The model under review builds one solid part; all positions refer to its coordinate system, in mm. A direction names the side the tool comes from. Coordinates: 2 decimals unless noted, no trailing zeros. Loops run counter-clockwise (first coordinate to the right, second up) from the corner with the lowest first, then second, coordinate; pieces in that order, holes last. Notation, with made-up numbers: M 51,61 L 88,61 A33 ccw 88,98 Z; hole C -28.75,-31.75 d2. An arc over 180 degrees is marked long. Use one line per item in the form item = value.
Autodesk Fusion 360 part; units mm, degrees
sketch "Sketch1" plane through (0, 0, 0) normal (0, 1, 0) x (1, 0, 0)
  line L0 (26, 0) -> (-26, 0)
  line L1 (0, 0) -> (0, -40) construction
  circle A0 centre (0, -20) radius 14
  circle A1 centre (0, -20) radius 19 construction
  line L2 (-26, 0) -> (-26, -28)
  line L3 (-26, -28) -> (-14, -40)
  line L4 (-14, -40) -> (14, -40)
  line L5 (14, -40) -> (26, -28)
  line L6 (26, -28) -> (26, 0)
  line L7 (26, -20) -> (-26, -20) construction
  line L8 (0, -20) -> (13.435, -33.435) construction
  line L9 (0, -20) -> (19, -20) construction
  line L10 (0, -20) -> (13.435, -6.565) construction
  line L11 (0, -20) -> (19, -20) construction
  line L12 (0, -20) -> (-13.435, -33.435) construction
  line L13 (0, -20) -> (19, -20) construction
  line L14 (0, -20) -> (-13.435, -6.565) construction
  line L15 (0, -20) -> (19, -20) construction
  circle A2 centre (-13.435, -33.435) radius 2.5
  circle A3 centre (-19, -20) radius 2.5
  circle A4 centre (-13.435, -6.565) radius 2.5
  circle A5 centre (13.435, -33.435) radius 2.5
  circle A6 centre (13.435, -6.565) radius 2.5
  circle A7 centre (19, -20) radius 2.5
  point P0 (0, -20)
  dimension "d2" = 52
  dimension "d3" = 40
  dimension "d4" = 28
  dimension "d5" = 38
  dimension "d6" = 135
  dimension "d8" = 135
  dimension "d10" = 12
  dimension "d12" = 45
  dimension "d13" = 45
  dimension "d16" = 45
  dimension "d17" = 45
  dimension "d18" = 5
  dimension "d19" = 5
  dimension "d20" = 5
  dimension "d21" = 5
  dimension "d23" = 5
  dimension "d27" = 5
  dimension "d28" = 19
extrude "Extrude1" add sketch "Sketch1" along normal blind 40 contours L0 L2 L3 L4 L5 L6 | A2 | A3 | A4 | A5 | A6 | A7
hole "Hole1" at (-19, 0, 20) at (-13.435, 0, 33.435) at (13.435, 0, 33.435) at (19, 0, 20) at (13.435, 0, 6.565) at (-13.435, 0, 6.565) direction (0, 1, 0) diameter 4.234 depth 15 tip angle 120 countersink diameter 5 countersink angle 90
sketch "Sketch2" plane through (0, 0, 0) normal (0, 0, -1) x (1, 0, 0)
  line L0 (26, 0) -> (-26, 0)
  line L1 (-26, 0) -> (-26, -40)
  line L2 (-26, -40) -> (26, -40)
  line L3 (26, -40) -> (26, 0)
  line L4 (-20, 0) -> (-20, -40) construction
  line L5 (0, 0) -> (0, -40) construction
  circle A0 centre (-20, -8) radius 2.5
  circle A1 centre (-20, -24) radius 2.5
  line L6 (-20, -20) -> (0, -20) construction
  circle A2 centre (20, -8) radius 2.5
  circle A3 centre (20, -24) radius 2.5
  dimension "d37" = 5
  dimension "d38" = 5
  dimension "d41" = 8
  dimension "d42" = 20
  dimension "d43" = 24
hole "Hole2" at (-20, 8, 0) at (-20, 24, 0) at (20, 8, 0) at (20, 24, 0) direction (0, 0, 1) diameter 4.234 depth 15 tip angle 120 countersink diameter 5.5 countersink angle 90
1. Wall thickness on line 1 along Y through (x, z) = (-20, 10); line 2 along Z through (x, y) = (-15, 10); line 3 along X through (y, z) = (24, 8): over which ranges is each line inside the solid? List them lowest first. Write a range as from..to.
Response values:
line_1 = 0..5.88, 10.12..21.88, 26.12..40
line_2 = 0..5.14, 7.99..32.01, 34.86..39
line_3 = -26..-22.12, -17.88..-7.21, 7.21..17.88, 22.12..26
2. Machinability: for faces 5 (the face through (17.57, 7.79, 21.56)), 6 (the face through (17.9, 7.72, 7.92)), 7 (the face through (0, 20, 0)), which of the approach directions +Z, -Z, +X, -X, +Y, -Y give a long, thin tool a straight path to every point of the face, cutting with its end or side? Answer none if there is none.
Response values:
face_5 = -Y
face_6 = -Z
face_7 = -Z, +X, -X, +Y, -Y
3. Add section C-C (z = 24). State the section outline as (x, y) points.
Response values:
outline = M -26,0 L -13.42,0 L -13.42,40 L -26,40 Z; M 13.42,0 L 26,0 L 26,40 L 13.42,40 Z
4. Add section A-A (y = 18.5). State the section outline as (x, z) points.
Response values:
outline = M -26,0 L 26,0 L 26,28 L 14,40 L -14,40 L -26,28 Z; hole C 0,20 d28
5. Add section B-B (x = 0). State the section outline as (y, z) points.
Response values:
outline = M 0,0 L 40,0 L 40,6 L 0,6 Z; M 0,34 L 40,34 L 40,40 L 0,40 Z
6. The part is to be moulded in two halves that separate along X. For faces 1 (the face through (-20, 20, 34)), 2 (the face through (-6, 40, 6)), 3 (the face through (18.57, 22.44, 7.92)), 4 (the face through (13.21, 16.01, 33.73)), say which applies: pulls with the +X half, pulls with the -X half, needs draft (parallel to the pull), parting line crosses it, or undercut.
Response values:
face_1 = pulls with the -X half
face_2 = needs draft
face_3 = undercut
face_4 = undercut
7. Add section D-D (z = 8). Count the separate pieces of the cut face and the enclosed holes in it, then the cut area to 3 significant figures.
Response values:
separate_pieces = 2
enclosed_holes = 4
area = 1,350 mm^2
8. Insertion check: P1, Ø2.5, axis at x = 13.435, z = 33.435, coming from the -Y side; P2, Ø3.5, axis at x = 20, y = 8, coming from the -Z side; P3, Ø5.5, axis at x = -20, y = 24, coming from the +Z side. Each pin has a flat end and moves straight along its axis. Give the tip position at first contact, or say it passes through.
Response values:
P1 = 15.5
P2 = 15.21
P3 = 36.75
